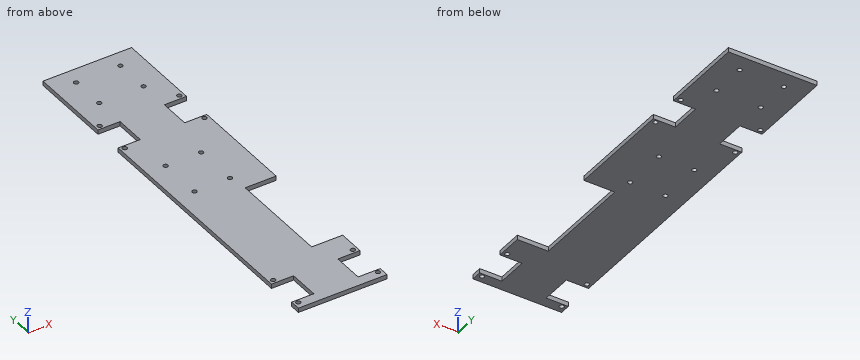
```python
from build123d import *

# Parameters (mm, degrees)
EXTRUDE_1_DEPTH     = 3
SKETCH_4_W          = 15
SKETCH_4_H          = 21
CUT_EXTRUDE_1_DEPTH = 3
SKETCH_5_R          = 1.55
CUT_EXTRUDE_2_DEPTH = 272.724124803
SKETCH_7_W          = 21
SKETCH_7_H          = 69
CUT_EXTRUDE_3_DEPTH = 272.724124803


with BuildPart() as part:
    # 草图1 → 凸台-拉伸1 (new body)
    with BuildSketch(Plane.XY):
        Polygon((0, 240), (0, 265), (60, 265), (60, 240), (60, 0), (0, 0), align=None)
    extrude(amount=EXTRUDE_1_DEPTH)

    # 草图4 → 切除-拉伸1 (cut)
    with BuildSketch(Plane(origin=(0, 0, 0), x_dir=(-1, 0, 0), z_dir=(0, 0, -1))):
        with Locations((-52.5, 17.5)):
            Rectangle(SKETCH_4_W, SKETCH_4_H)
        with Locations((-7.5, 17.5)):
            Rectangle(SKETCH_4_W, SKETCH_4_H)
        with Locations((-7.5, 197.5)):
            Rectangle(SKETCH_4_W, SKETCH_4_H)
        with Locations((-52.5, 197.5)):
            Rectangle(SKETCH_4_W, SKETCH_4_H)
    extrude(amount=-CUT_EXTRUDE_1_DEPTH, mode=Mode.SUBTRACT)

    # 草图5 → 切除-拉伸2 (cut, through all)
    with BuildSketch(Plane(origin=(0, 0, 0), x_dir=(-1, 0, 0), z_dir=(0, 0, -1))):
        with Locations((-45, 229.6)):
            Circle(SKETCH_5_R)
        with Locations((-45, 253.6)):
            Circle(SKETCH_5_R)
        with Locations((-15, 253.6)):
            Circle(SKETCH_5_R)
        with Locations((-15, 229.6)):
            Circle(SKETCH_5_R)
        with Locations((-57, 184.75)):
            Circle(SKETCH_5_R)
        with Locations((-3, 184.75)):
            Circle(SKETCH_5_R)
        with Locations((-3, 210.85)):
            Circle(SKETCH_5_R)
        with Locations((-57, 210.85)):
            Circle(SKETCH_5_R)
        with Locations((-13, 127.7)):
            Circle(SKETCH_5_R)
        with Locations((-37, 127.7)):
            Circle(SKETCH_5_R)
        with Locations((-37, 157.7)):
            Circle(SKETCH_5_R)
        with Locations((-13, 157.7)):
            Circle(SKETCH_5_R)
        with Locations((-57, 4.75)):
            Circle(SKETCH_5_R)
        with Locations((-3, 4.75)):
            Circle(SKETCH_5_R)
        with Locations((-3, 30.85)):
            Circle(SKETCH_5_R)
        with Locations((-57, 30.85)):
            Circle(SKETCH_5_R)
    extrude(amount=-CUT_EXTRUDE_2_DEPTH, mode=Mode.SUBTRACT)

    # 草图7 → 切除-拉伸3 (cut, through all)
    with BuildSketch(Plane(origin=(0, 0, 0), x_dir=(-1, 0, 0), z_dir=(0, 0, -1))):
        with Locations((-49.5, 80.5)):
            Rectangle(SKETCH_7_W, SKETCH_7_H)
    extrude(amount=-CUT_EXTRUDE_3_DEPTH, mode=Mode.SUBTRACT)


solid = part.part
```
Verification items for the finished model (mm, model axes). Round coordinates to 2 decimals unless told otherwise and drop trailing zeros. Order: outer loops, then holes, each group sorted by start corner. A loop starts at its lowest first (then second) coordinate and runs counter-clockwise, first axis right, second up. Notation, with made-up numbers: (35.25, 73.5) -> (48.25, 73.5) arc R14 ccw to (48.25, 85.5) -> close; hole circle Ø7 at (26.25, 61). An arc over 180 degrees is marked (long way). Put each result on its own line as item: value. Start each with the question number.
(1) Section check A-A (z = 1.8). State how many separate pieces and enclosed holes the cut face has, then the cut area to 3 significant figures.
(2) Section check B-B (y = 57.5). Enter the section's corners in (x, z), then the cut area to 3 significant figures.
(3) Material ranges on line 1 along X through (y, z) = (184.75, 1); line 2 along X through (y, z) = (253.6, 1.3); line 3 along Y through (x, z) = (13, 1.9), recorded low to high.
(4) Depth check by flat-ended pin: pin 1 Ø3 at (x, y) = (57, 210.85) entering from -Z. Enter the tip coordinate at first touch or a pass-through.
Completed:
1. separate pieces: 1
1. enclosed holes: 16
1. area: 13,100 mm2
2. outline: (0, 0) -> (39, 0) -> (39, 3) -> (0, 3) -> close
2. area: 117 mm2
3. line 1: x = 0 to 1.45, 4.55 to 55.45, 58.55 to 60
3. line 2: x = 0 to 13.45, 16.55 to 43.45, 46.55 to 60
3. line 3: y = 0 to 7, 28 to 126.15, 129.25 to 156.15, 159.25 to 187, 208 to 265
4. pin 1: passes through
